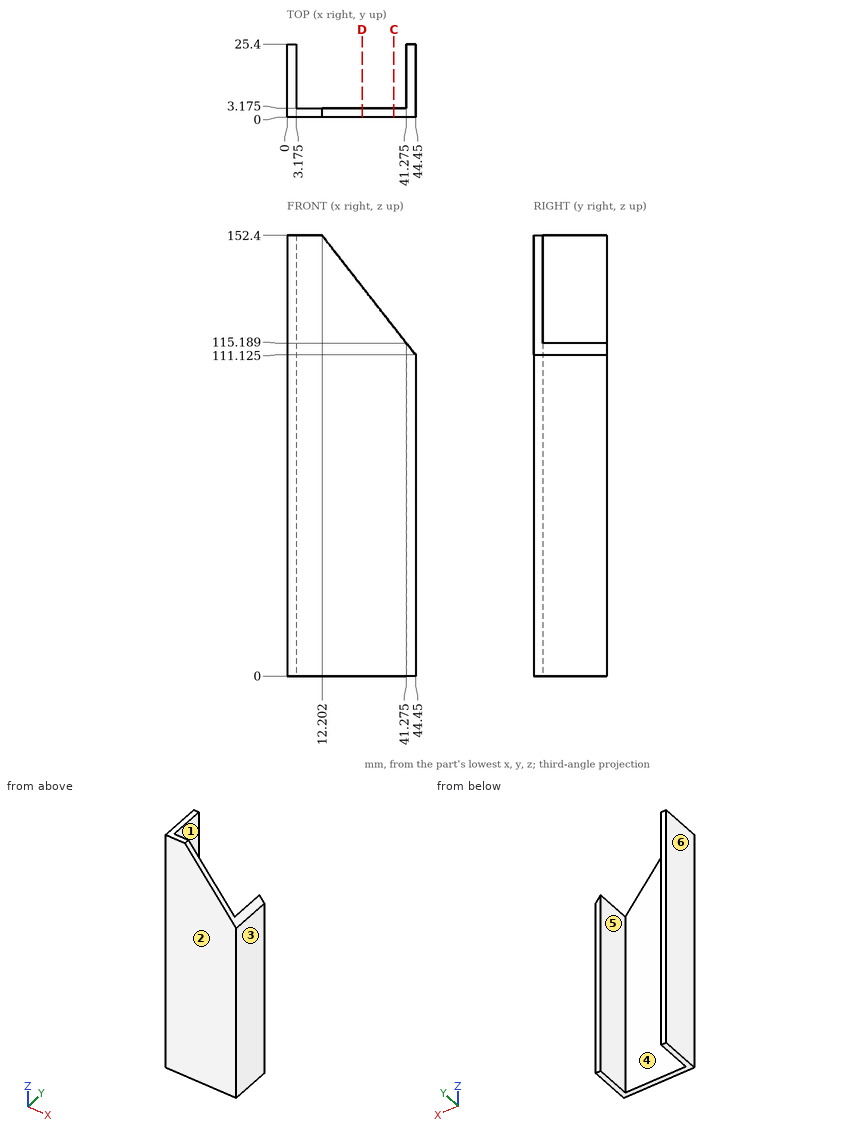
Geometry check sheet. Reference: drawing and pictorial views, mm from the part's lowest x, y, z. A direction names the side the tool comes from. Round coordinates to 2 decimals unless told otherwise and drop trailing zeros. Order: outer loops, then holes, each group sorted by start corner. A loop starts at its lowest first (then second) coordinate and runs counter-clockwise, first axis right, second up. Notation, with made-up numbers: M 33,-38 L 80,-38 A20 ccw 80,-29 Z; hole C 42,45.25 d3. An arc over 180 degrees is marked long. One line per item, written item: value. Start each with the question number.
1. Gauge pin test, flat end, axial feed: P1, Ø4, axis at x = 6.5, z = 109.5, coming from the +Y side (3 decimals). Record the tip position at first contact, or that the pin passes through.
2. Section check D-D on x = 26. Enter the section's corners in (y, z) (1 decimal).
3. Section check C-C on x = 37. Enter the section's corners in (y, z) (1 decimal), and give its area (3 significant figures).
4. Scan lines: line 1 along Y through (x, z) = (39.5, 41) (1 decimal); line 2 along X through (y, z) = (2.25, 139). Record each from-to range of solid material in increasing order.
5. Release check for a two-part mould opening along X. For the marked faces 1, 2, 3 and 4 record: released by +X, released by -X, zero draft, split by the parting line, or undercut.
6. Access from +Z, -Z, +X, -X, +Y, -Y to the whole of each face (thin tool, end or side, straight path). Record for the marked faces 5 and 6.
Results found:
1. P1: y = 3.175
2. outline: M 0,0 L 3.2,0 L 3.2,134.7 L 0,134.7 Z
3. outline: M 0,0 L 3.2,0 L 3.2,120.7 L 0,120.7 Z
3. area: 383 mm^2
4. line 1: 0 to 3.2
4. line 2: 0 to 22.67
5. face 1: undercut
5. face 2: zero draft
5. face 3: released by +X
5. face 4: undercut
6. face 5: +Z, -Z, +Y
6. face 6: +Z, -Z, -X, +Y, -Y
